```python
from build123d import *

# Parameters (mm, degrees)
F0_W            = 107.95
F0_H            = 69.85
F1_DEPTH        = 22.225
F2_W            = 50.8
F2_H            = 3.048
F2_W_2          = 38.1
F3_DEPTH        = 22.226
F3_DEPTH_BACK   = 22.226
F4_W            = 19.05
F4_H            = 6.096
F5_DEPTH        = 53.976
F5_DEPTH_BACK   = 53.976
F7_DEPTH        = 25.4
F8_R            = 119.126
F9_DEPTH        = 7.874
F10_R           = 76.2
F11_DEPTH       = 7.874
F14_D           = 12.7
F14_CBORE_D     = 19.05
F14_CBORE_DEPTH = 20.574
F15_D           = 12.7
F16_R           = 9.525
F17_DEPTH       = 20.574
F18_SIZE2       = 9.0921120392
F18_SIZE        = 15.748


with BuildPart() as f1:
    # F0 (on Front) → F1 (new body, symmetric)
    with BuildSketch(Plane.XZ):
        Rectangle(F0_W, F0_H)
    extrude(amount=F1_DEPTH, both=True)

    # F2 (on Front) → F3 (cut, two sides)
    with BuildSketch(Plane.XZ) as f3_sk:
        with Locations((-28.575, -33.401)):
            Rectangle(F2_W, F2_H)
        with Locations((34.925, -33.401)):
            Rectangle(F2_W_2, F2_H)
    extrude(amount=-F3_DEPTH, mode=Mode.SUBTRACT)
    extrude(f3_sk.sketch, amount=F3_DEPTH_BACK, mode=Mode.SUBTRACT)

    # F4 (on Right) → F5 (cut, two sides)
    with BuildSketch(Plane.YZ) as f5_sk:
        with Locations((0, -31.877)):
            Rectangle(F4_W, F4_H)
    extrude(amount=F5_DEPTH, mode=Mode.SUBTRACT)
    extrude(f5_sk.sketch, amount=-F5_DEPTH_BACK, mode=Mode.SUBTRACT)

    # F6 (on face) → F7 (cut)
    with BuildSketch(Plane.XY.offset(34.925)):
        with BuildLine():
            Line((53.975, 22.225), (-9.525, 22.225))
            ThreePointArc((-9.525, 22.225), (-11.7065832479, 0), (-9.525, -22.225))
            Line((-9.525, -22.225), (53.975, -22.225))
            Line((53.975, -22.225), (53.975, 22.225))
        make_face()
    extrude(amount=-F7_DEPTH, mode=Mode.SUBTRACT)

    # F8 (on face) → F9 (cut)
    with BuildSketch(Plane.XY.offset(9.525)):
        with Locations((102.5934167521, 0)):
            Circle(F8_R)
    extrude(amount=-F9_DEPTH, mode=Mode.SUBTRACT)

    # F10 (on face) → F11 (cut)
    with BuildSketch(Plane.XY.offset(1.651)):
        with Locations((102.5934167521, 0)):
            Circle(F10_R)
    extrude(amount=-F11_DEPTH, mode=Mode.SUBTRACT)

    # F14 (through all)
    with Locations(Plane.XY.offset(34.925)):
        with Locations((-28.575, 0)):
            CounterBoreHole(F14_D / 2, F14_CBORE_D / 2, F14_CBORE_DEPTH)

    # F15 (through all)
    with Locations(Plane.XY.offset(1.651)):
        with Locations((34.925, 0)):
            Hole(F15_D / 2)

    # F16 (on face) → F17 (cut)
    with BuildSketch(Plane.XY.offset(1.651)):
        with Locations((34.925, 0)):
            Circle(F16_R)
    extrude(amount=-F17_DEPTH, mode=Mode.SUBTRACT)

    # F18
    f18_edges = [f1.edges().sort_by_distance(p)[0] for p in [
        (-53.975, 0, 34.925),
    ]]
    f18_side = f1.faces().sort_by_distance((-53.975, 0, 2.159774))[0]
    chamfer(f18_edges, length=F18_SIZE, length2=F18_SIZE2, reference=f18_side)


solid = f1.part
```
Could you check a few things on this model? Use its own coordinates, in mm. A direction names the side the tool comes from. Give positions to 0.01 mm unless a question says otherwise; leave off trailing zeros. Loops run counter-clockwise (first coordinate to the right, second up) from the corner with the lowest first, then second, coordinate; pieces in that order, holes last. Notation, with made-up numbers: (45.5, 56.25) - (62.5, 56.25) arc R14 cw to (62.5, 73.25) - close; hole circle Ø4 at (-37.75, -2). An arc over 180 degrees is marked (long way). Use one line per item in the form item = value.
1. I want a section at C-C (z = 11.5). Please give me the cut outline in (x, y) (3 decimals), and give its area (3 significant figures).
Response values:
outline = (-53.975, -22.225) - (-9.525, -22.225) arc R114.3 cw to (-9.525, 22.225) - (-53.975, 22.225) - close; hole circle Ø12.7 at (-28.575, 0)
area = 1,780 mm²
2. Thinking about a two-plate mould opening in Y: for faces 4 (the face through (1, 0, -28.829)), 5 (the face through (-13, 22.225, -7)), 6 (the face through (-20, -5, 34.925)), which applies, released by +Y, released by -Y, zero draft, split by the parting line, or undercut?
Response values:
face_4 = undercut
face_5 = released by +Y
face_6 = zero draft
3. On a 3-axis mill with a long thin cutter (end or side, diameter ignored), from which of +Z, -Z, +X, -X, +Y, -Y can I reach the whole of each face in a straight line? I mean faces 1 (the face through (-13, 0, 9.525)), 2 (the face through (35, 16, -31.877)), 3 (the face through (27.57, -13.33, -2.23)). Say none if no direction works.
Response values:
face_1 = +X
face_2 = -Z, +X, +Y, -Y
face_3 = +Z, +X
4. I want a section at D-D (y = -19). Please give me the cut outline in (x, z) (3 decimals).
Response values:
outline = (-53.975, -31.877) - (-3.175, -31.877) - (-3.175, -34.925) - (15.875, -34.925) - (15.875, -31.877) - (53.975, -31.877) - (53.975, -6.223) - (28.8, -6.223) - (28.8, 1.651) - (-15.008, 1.651) - (-15.008, 9.525) - (-10.116, 9.525) - (-10.116, 34.925) - (-44.883, 34.925) - (-53.975, 19.177) - close
5. I want a section at B-B (x = 20). Please give me the cut outline in (y, z) (3 decimals).
Response values:
outline = (-22.225, -31.877) - (-9.525, -31.877) - (-9.525, -28.829) - (9.525, -28.829) - (9.525, -31.877) - (22.225, -31.877) - (22.225, 1.651) - (-22.225, 1.651) - close
6. I want a section at A-A (y = 0). Please give me the cut outline in (x, z) (3 decimals), and give its area (3 significant figures).
Response values:
outline = (-53.975, -28.829) - (-34.925, -28.829) - (-34.925, 14.351) - (-38.1, 14.351) - (-38.1, 34.925) - (-44.883, 34.925) - (-53.975, 19.177) - close; (-22.225, -28.829) - (28.575, -28.829) - (28.575, -18.923) - (25.4, -18.923) - (25.4, 1.651) - (-16.533, 1.651) - (-16.533, 9.525) - (-11.707, 9.525) - (-11.707, 34.925) - (-19.05, 34.925) - (-19.05, 14.351) - (-22.225, 14.351) - close; (41.275, -28.829) - (53.975, -28.829) - (53.975, -6.223) - (44.45, -6.223) - (44.45, -18.923) - (41.275, -18.923) - close
area = 3,050 mm²
7. I need wall thicknesses on probe 1 along Y at (x, z) = (-28.5, 29) (3 decimals); probe 2 along Z at (x, y) = (25, 5); probe 3 along Z at (x, y) = (-21, -5). Which ranges of each line are inside material? Lowest first, please.
Response values:
probe_1 = -22.225 to -9.525, 9.525 to 22.225
probe_2 = -28.83 to 1.65
probe_3 = -28.83 to 14.35
8. I'm going to push flat-ended pins straight in: pin 1 Ø17 at (x, y) = (-28.575, 0) entering from -Z; pin 2 Ø3 at (y, z) = (4.5, 16) entering from +X; pin 3 Ø13.5 at (x, y) = (9, -7.5) entering from +Z; pin 4 Ø5.5 at (x, y) = (35, 2) entering from +Z. Where does each tip first touch, or does it pass through?
Response values:
pin_1 = -28.83
pin_2 = -11.55
pin_3 = 1.65
pin_4 = through
